Check sheet for the modelled part. Datum: model origin and axes. Units: mm. A direction names the side the tool comes from. Give positions to 0.01 mm unless a question says otherwise; leave off trailing zeros. Order: outer loops, then holes, each group sorted by start corner. A loop starts at its lowest first (then second) coordinate and runs counter-clockwise, first axis right, second up.
from build123d import *

# Parameters (mm, degrees)
SKETCH1_R           = 5
BOSS_EXTRUDE4_DEPTH = 5
SKETCH4_W           = 40
SKETCH4_H           = 5
BOSS_EXTRUDE5_DEPTH = 20
BOSS_EXTRUDE6_START = 5
SKETCH5_R           = 5
BOSS_EXTRUDE6_DEPTH = 5
SKETCH7_R           = 2
CUT_EXTRUDE1_DEPTH  = 15


with BuildPart() as part:
    # Sketch1 → Boss-Extrude4 (new body)
    with BuildSketch(Plane.XY):
        with BuildLine():
            Line((-20, -35), (20, -35))
            Line((20, -35), (20, 5))
            ThreePointArc((20, 5), (17.071067812, 12.071067812), (10, 15))
            Line((10, 15), (-10, 15))
            ThreePointArc((-10, 15), (-17.071067812, 12.071067812), (-20, 5))
            Line((-20, 5), (-20, -35))
        make_face()
        Circle(SKETCH1_R, mode=Mode.SUBTRACT)
    extrude(amount=BOSS_EXTRUDE4_DEPTH)

    # Sketch4 → Boss-Extrude5 (add)
    with BuildSketch(Plane(origin=(0, 0, 0), x_dir=(-1, 0, 0), z_dir=(0, 0, -1))):
        with Locations((0, -32.5)):
            Rectangle(SKETCH4_W, SKETCH4_H)
    extrude(amount=BOSS_EXTRUDE5_DEPTH)

    # Sketch5 → Boss-Extrude6 (add)
    with BuildSketch(Plane(origin=(0, 0, -20), x_dir=(-1, 0, 0), z_dir=(0, 0, -1)).offset(BOSS_EXTRUDE6_START)):
        with BuildLine():
            Line((-20, 5), (-20, -35))
            Line((-20, -35), (20, -35))
            Line((20, -35), (20, -30))
            Line((20, -30), (20, 5))
            ThreePointArc((20, 5), (17.071067812, 12.071067812), (10, 15))
            Line((10, 15), (-10, 15))
            ThreePointArc((-10, 15), (-17.071067812, 12.071067812), (-20, 5))
        make_face()
        with Locations(Location((0, 0, 0), (0, 0, 180))):
            Circle(SKETCH5_R, mode=Mode.SUBTRACT)
    extrude(amount=-BOSS_EXTRUDE6_DEPTH)

    # Sketch7 → Cut-Extrude1 (cut)
    with BuildSketch(Plane(origin=(0, -30, 0), x_dir=(1, 0, 0), z_dir=(0, 1, 0))):
        with Locations(Location((-7, 10, 0), (0, 0, 270))):
            Circle(SKETCH7_R)
        with Locations(Location((7, 10, 0), (0, 0, 270))):
            Circle(SKETCH7_R)
    extrude(amount=-CUT_EXTRUDE1_DEPTH, mode=Mode.SUBTRACT)


solid = part.part
1) Set-up check for faces 5 (the face through (0, -7, 0)), 6 (the face through (20, -19.2, -20.2)): record each of +Z, -Z, +X, -X, +Y, -Y from which the full face is reachable in a straight line by a thin tool's end or side.
Recorded:
face 5: +X, -X, +Y
face 6: +Z, -Z, +X, +Y, -Y
2) Section check B-B, the plane y = -12. Record the cut outline in (x, z).
Recorded:
outline: (-20, -25) - (20, -25) - (20, -20) - (-20, -20) - close; (-20, 0) - (20, 0) - (20, 5) - (-20, 5) - close
3) Section check A-A, the plane z = -10. Record the cut outline in (x, y).
Recorded:
outline: (-20, -35) - (-9, -35) - (-9, -30) - (-20, -30) - close; (-5, -35) - (5, -35) - (5, -30) - (-5, -30) - close; (9, -35) - (20, -35) - (20, -30) - (9, -30) - close
4) Material ranges on L1, parallel to X at y = -32.1, z = -10; L2, parallel to Z at x = 5, y = -11; L3, parallel to Y at x = 0, z = -21.1, recorded low to high.
Recorded:
L1: x = -20 to -9, -5 to 5, 9 to 20
L2: z = -25 to -20, 0 to 5
L3: y = -35 to -5, 5 to 15
5) Depth check by flat-ended pin: pin 1 Ø12 at (x, y) = (-1, -3.5) entering from -Z; pin 2 Ø6 at (x, z) = (-5, -8) entering from +Y; pin 3 Ø1.5 at (y, z) = (-2.5, -18.5) entering from +X. Enter the tip coordinate at first touch or a pass-through.
Recorded:
pin 1: stops at z = -25
pin 2: stops at y = -30
pin 3: passes through
6) Section check D-D, the plane x = -7. Record the cut outline in (y, z).
Recorded:
outline: (-35, -25) - (15, -25) - (15, -20) - (-30, -20) - (-30, -12) - (-35, -12) - close; (-35, -8) - (-30, -8) - (-30, 0) - (15, 0) - (15, 5) - (-35, 5) - close
7) Draft check along X on faces 1 (the face through (-1.08, -4.88, 2.46)), 2 (the face through (-16.99, 12.15, 2.46)), 3 (the face through (0, 15, -23)), 4 (the face through (9, -32, -10)). Enter one of: +X half, -X half, draft (parallel to the pull), parting line (faces both ways), or undercut.
Recorded:
face 1: undercut
face 2: -X half
face 3: draft
face 4: undercut
8) Section check C-C, the plane x = 0. Record the cut outline in (y, z), then the cut area to 3 significant figures.
Recorded:
outline: (-35, -25) - (-5, -25) - (-5, -20) - (-30, -20) - (-30, 0) - (-5, 0) - (-5, 5) - (-35, 5) - close; (5, -25) - (15, -25) - (15, -20) - (5, -20) - close; (5, 0) - (15, 0) - (15, 5) - (5, 5) - close
area: 500 mm2
